```python
from build123d import *

# Parameters (mm, degrees)
BOX_SIDE_DEPTH       = 6
SKETCH2_R            = 1.5
SCREW_CUT_OUTS_DEPTH = 107.235587258


with BuildPart() as part:
    # Sketch1 → Box Side (new body)
    with BuildSketch(Plane.XY):
        Polygon((-69, 69), (-23, 69), (-23, 75), (23, 75), (23, 69), (69, 69), (69, 23), (75, 23), (75, -23), (69, -23), (69, -69), (69, -75), (23, -75), (23, -69), (-23, -69), (-23, -75), (-69, -75), (-75, -75), (-75, -69), (-75, -23), (-69, -23), (-69, 23), (-75, 23), (-75, 69), align=None)
    extrude(amount=BOX_SIDE_DEPTH)

    # Sketch2 → Screw Cut-outs (cut, through all)
    with BuildSketch(Plane.XY.offset(6)):
        with Locations((0, 72)):
            Circle(SKETCH2_R)
        with Locations(Location((72, 0, 0), (0, 0, 180))):
            Circle(SKETCH2_R)
        with Locations((-46, -72)):
            Circle(SKETCH2_R)
        with Locations(Location((46, -72, 0), (0, 0, 180))):
            Circle(SKETCH2_R)
        with Locations((-72, 46)):
            Circle(SKETCH2_R)
        with Locations(Location((-72, -46, 0), (0, 0, 180))):
            Circle(SKETCH2_R)
        with BuildLine():
            Line((-44.5, 69), (-44.5, 64.2))
            ThreePointArc((-44.5, 64.2), (-44.441421356, 64.058578644), (-44.3, 64))
            Line((-44.3, 64), (-42.7, 64))
            ThreePointArc((-42.7, 64), (-42.558578644, 63.941421356), (-42.5, 63.8))
            Line((-42.5, 63.8), (-42.5, 61.2))
            ThreePointArc((-42.5, 61.2), (-42.558578644, 61.058578644), (-42.7, 61))
            Line((-42.7, 61), (-44.3, 61))
            ThreePointArc((-44.3, 61), (-44.441421356, 60.941421356), (-44.5, 60.8))
            Line((-44.5, 60.8), (-44.5, 57.2))
            ThreePointArc((-44.5, 57.2), (-44.558578644, 57.058578644), (-44.7, 57))
            Line((-44.7, 57), (-47.3, 57))
            ThreePointArc((-47.3, 57), (-47.441421356, 57.058578644), (-47.5, 57.2))
            Line((-47.5, 57.2), (-47.5, 60.8))
            ThreePointArc((-47.5, 60.8), (-47.558578644, 60.941421356), (-47.7, 61))
            Line((-47.7, 61), (-49.3, 61))
            ThreePointArc((-49.3, 61), (-49.441421356, 61.058578644), (-49.5, 61.2))
            Line((-49.5, 61.2), (-49.5, 63.8))
            ThreePointArc((-49.5, 63.8), (-49.441421356, 63.941421356), (-49.3, 64))
            Line((-49.3, 64), (-47.7, 64))
            ThreePointArc((-47.7, 64), (-47.558578644, 64.058578644), (-47.5, 64.2))
            Line((-47.5, 64.2), (-47.5, 69))
            Line((-47.5, 69), (-44.5, 69))
        make_face()
        with BuildLine():
            Line((47.5, 69), (47.5, 64.2))
            ThreePointArc((47.5, 64.2), (47.558578644, 64.058578644), (47.7, 64))
            Line((47.7, 64), (49.3, 64))
            ThreePointArc((49.3, 64), (49.441421356, 63.941421356), (49.5, 63.8))
            Line((49.5, 63.8), (49.5, 61.2))
            ThreePointArc((49.5, 61.2), (49.441421356, 61.058578644), (49.3, 61))
            Line((49.3, 61), (47.7, 61))
            ThreePointArc((47.7, 61), (47.558578644, 60.941421356), (47.5, 60.8))
            Line((47.5, 60.8), (47.5, 57.2))
            ThreePointArc((47.5, 57.2), (47.441421356, 57.058578644), (47.3, 57))
            Line((47.3, 57), (44.7, 57))
            ThreePointArc((44.7, 57), (44.558578644, 57.058578644), (44.5, 57.2))
            Line((44.5, 57.2), (44.5, 60.8))
            ThreePointArc((44.5, 60.8), (44.441421356, 60.941421356), (44.3, 61))
            Line((44.3, 61), (42.7, 61))
            ThreePointArc((42.7, 61), (42.558578644, 61.058578644), (42.5, 61.2))
            Line((42.5, 61.2), (42.5, 63.8))
            ThreePointArc((42.5, 63.8), (42.558578644, 63.941421356), (42.7, 64))
            Line((42.7, 64), (44.3, 64))
            ThreePointArc((44.3, 64), (44.441421356, 64.058578644), (44.5, 64.2))
            Line((44.5, 64.2), (44.5, 69))
            Line((44.5, 69), (47.5, 69))
        make_face()
        with BuildLine():
            Line((69, 44.5), (64.2, 44.5))
            ThreePointArc((64.2, 44.5), (64.058578644, 44.441421356), (64, 44.3))
            Line((64, 44.3), (64, 42.7))
            ThreePointArc((64, 42.7), (63.941421356, 42.558578644), (63.8, 42.5))
            Line((63.8, 42.5), (61.2, 42.5))
            ThreePointArc((61.2, 42.5), (61.058578644, 42.558578644), (61, 42.7))
            Line((61, 42.7), (61, 44.3))
            ThreePointArc((61, 44.3), (60.941421356, 44.441421356), (60.8, 44.5))
            Line((60.8, 44.5), (57.2, 44.5))
            ThreePointArc((57.2, 44.5), (57.058578644, 44.558578644), (57, 44.7))
            Line((57, 44.7), (57, 47.3))
            ThreePointArc((57, 47.3), (57.058578644, 47.441421356), (57.2, 47.5))
            Line((57.2, 47.5), (60.8, 47.5))
            ThreePointArc((60.8, 47.5), (60.941421356, 47.558578644), (61, 47.7))
            Line((61, 47.7), (61, 49.3))
            ThreePointArc((61, 49.3), (61.058578644, 49.441421356), (61.2, 49.5))
            Line((61.2, 49.5), (63.8, 49.5))
            ThreePointArc((63.8, 49.5), (63.941421356, 49.441421356), (64, 49.3))
            Line((64, 49.3), (64, 47.7))
            ThreePointArc((64, 47.7), (64.058578644, 47.558578644), (64.2, 47.5))
            Line((64.2, 47.5), (69, 47.5))
            Line((69, 47.5), (69, 44.5))
        make_face()
        with BuildLine():
            Line((69, -47.5), (64.2, -47.5))
            ThreePointArc((64.2, -47.5), (64.058578644, -47.558578644), (64, -47.7))
            Line((64, -47.7), (64, -49.3))
            ThreePointArc((64, -49.3), (63.941421356, -49.441421356), (63.8, -49.5))
            Line((63.8, -49.5), (61.2, -49.5))
            ThreePointArc((61.2, -49.5), (61.058578644, -49.441421356), (61, -49.3))
            Line((61, -49.3), (61, -47.7))
            ThreePointArc((61, -47.7), (60.941421356, -47.558578644), (60.8, -47.5))
            Line((60.8, -47.5), (57.2, -47.5))
            ThreePointArc((57.2, -47.5), (57.058578644, -47.441421356), (57, -47.3))
            Line((57, -47.3), (57, -44.7))
            ThreePointArc((57, -44.7), (57.058578644, -44.558578644), (57.2, -44.5))
            Line((57.2, -44.5), (60.8, -44.5))
            ThreePointArc((60.8, -44.5), (60.941421356, -44.441421356), (61, -44.3))
            Line((61, -44.3), (61, -42.7))
            ThreePointArc((61, -42.7), (61.058578644, -42.558578644), (61.2, -42.5))
            Line((61.2, -42.5), (63.8, -42.5))
            ThreePointArc((63.8, -42.5), (63.941421356, -42.558578644), (64, -42.7))
            Line((64, -42.7), (64, -44.3))
            ThreePointArc((64, -44.3), (64.058578644, -44.441421356), (64.2, -44.5))
            Line((64.2, -44.5), (69, -44.5))
            Line((69, -44.5), (69, -47.5))
        make_face()
        with BuildLine():
            Line((-1.5, -69), (1.5, -69))
            Line((1.5, -69), (1.5, -64.2))
            ThreePointArc((1.5, -64.2), (1.558578644, -64.058578644), (1.7, -64))
            Line((1.7, -64), (3.3, -64))
            ThreePointArc((3.3, -64), (3.441421356, -63.941421356), (3.5, -63.8))
            Line((3.5, -63.8), (3.5, -61.2))
            ThreePointArc((3.5, -61.2), (3.441421356, -61.058578644), (3.3, -61))
            Line((3.3, -61), (1.7, -61))
            ThreePointArc((1.7, -61), (1.558578644, -60.941421356), (1.5, -60.8))
            Line((1.5, -60.8), (1.5, -57.2))
            ThreePointArc((1.5, -57.2), (1.441421356, -57.058578644), (1.3, -57))
            Line((1.3, -57), (-1.3, -57))
            ThreePointArc((-1.3, -57), (-1.441421356, -57.058578644), (-1.5, -57.2))
            Line((-1.5, -57.2), (-1.5, -60.8))
            ThreePointArc((-1.5, -60.8), (-1.558578644, -60.941421356), (-1.7, -61))
            Line((-1.7, -61), (-3.3, -61))
            ThreePointArc((-3.3, -61), (-3.441421356, -61.058578644), (-3.5, -61.2))
            Line((-3.5, -61.2), (-3.5, -63.8))
            ThreePointArc((-3.5, -63.8), (-3.441421356, -63.941421356), (-3.3, -64))
            Line((-3.3, -64), (-1.7, -64))
            ThreePointArc((-1.7, -64), (-1.558578644, -64.058578644), (-1.5, -64.2))
            Line((-1.5, -64.2), (-1.5, -69))
        make_face()
        with BuildLine():
            Line((-69, -1.5), (-64.2, -1.5))
            ThreePointArc((-64.2, -1.5), (-64.058578644, -1.558578644), (-64, -1.7))
            Line((-64, -1.7), (-64, -3.3))
            ThreePointArc((-64, -3.3), (-63.941421356, -3.441421356), (-63.8, -3.5))
            Line((-63.8, -3.5), (-61.2, -3.5))
            ThreePointArc((-61.2, -3.5), (-61.058578644, -3.441421356), (-61, -3.3))
            Line((-61, -3.3), (-61, -1.7))
            ThreePointArc((-61, -1.7), (-60.941421356, -1.558578644), (-60.8, -1.5))
            Line((-60.8, -1.5), (-57.2, -1.5))
            ThreePointArc((-57.2, -1.5), (-57.058578644, -1.441421356), (-57, -1.3))
            Line((-57, -1.3), (-57, 1.3))
            ThreePointArc((-57, 1.3), (-57.058578644, 1.441421356), (-57.2, 1.5))
            Line((-57.2, 1.5), (-60.8, 1.5))
            ThreePointArc((-60.8, 1.5), (-60.941421356, 1.558578644), (-61, 1.7))
            Line((-61, 1.7), (-61, 3.3))
            ThreePointArc((-61, 3.3), (-61.058578644, 3.441421356), (-61.2, 3.5))
            Line((-61.2, 3.5), (-63.8, 3.5))
            ThreePointArc((-63.8, 3.5), (-63.941421356, 3.441421356), (-64, 3.3))
            Line((-64, 3.3), (-64, 1.7))
            ThreePointArc((-64, 1.7), (-64.058578644, 1.558578644), (-64.2, 1.5))
            Line((-64.2, 1.5), (-69, 1.5))
            Line((-69, 1.5), (-69, -1.5))
        make_face()
    extrude(amount=-SCREW_CUT_OUTS_DEPTH, mode=Mode.SUBTRACT)


solid = part.part
```
The listing builds one solid part. Answer for the finished solid, in the listing's coordinates (mm). A direction names the side the tool comes from. Round coordinates to 2 decimals unless told otherwise and drop trailing zeros. Write each loop counter-clockwise with the first axis right and the second up, starting at its lowest first coordinate (ties: lowest second). Pieces come first, ordered by that corner, then holes. Notation, with made-up numbers: (62, 56) -> (98, 56) arc R29 cw to (98, 91) -> close; hole circle Ø10 at (58.5, 9). An arc over 180 degrees is marked (long way). Answer as a JSON object with one key per item and string values. Group by question number.
Q1. Section B-B (x = -7) is taken. Write down the section's boundary in (y, z).
Q2. Determine the mould class of faces 1 (the face through (47.5, 59, 3)), 2 (the face through (-34, 69, 3)), 3 (the face through (69, -61, 3)), 4 (the face through (-1.5, -59, 3)) for opening direction X: pulls with the +X half, pulls with the -X half, needs draft (parallel to the pull), parting line crosses it, or undercut.
Q3. Section A-A (z = 4.3) is taken. Count the separate pieces of the cut face and the enclosed holes in it, plus the area to 3 significant figures.
Q4. Each of these flat-tipped pins is pushed along its axis until it touches: pin 1 Ø0.8 at (y, z) = (0, 2) entering from -X; pin 2 Ø3 at (y, z) = (38.5, 2.5) entering from +X; pin 3 Ø0.5 at (x, z) = (-2, 1.5) entering from -Y; pin 4 Ø3.5 at (x, y) = (72, 0) entering from -Z. Where does it stop, or does it pass through?
Q5. Which of the six approach directions +Z, -Z, +X, -X, +Y, -Y give full straight-line access (tool end or side, diameter ignored) to faces 5 (the face through (12, -69, 3)), 6 (the face through (47.5, 67, 3)), 7 (the face through (34, 69, 3)), 8 (the face through (59, 44.5, 3)), 9 (the face through (1, 1, 6))?
Q6. Straight lines are drawn through the part: line 1 along Y through (x, z) = (-72, 3.45); line 2 along X through (y, z) = (61.5, 5.4). For each, find the intervals that lie inside material, in ascending order.
Check values:
{
 "1": {"outline": "(-69, 0) -> (75, 0) -> (75, 6) -> (-69, 6) -> close"},
 "2": {"face 1": "undercut", "face 2": "needs draft", "face 3": "pulls with the +X half", "face 4": "undercut"},
 "3": {"separate pieces": "1", "enclosed holes": "6", "area": "20,400 mm^2"},
 "4": {"pin 1": "x = -57", "pin 2": "x = 69", "pin 3": "y = -69", "pin 4": "z = 0"},
 "5": {"face 5": "+Z, -Z, -Y", "face 6": "+Z, -Z, +Y", "face 7": "+Z, -Z, +X, +Y", "face 8": "+Z, -Z, +X", "face 9": "+Z, +X, -X, +Y, -Y"},
 "6": {"line 1": "-75 to -47.5, -44.5 to -23, 23 to 44.5, 47.5 to 69", "line 2": "-75 to -49.5, -42.5 to 42.5, 49.5 to 69"}
}
